Part model, mm, in its own coordinate system. A direction names the side the tool comes from. Coordinates: 2 decimals unless noted, no trailing zeros. Write each loop counter-clockwise with the first axis right and the second up, starting at its lowest first coordinate (ties: lowest second). Pieces come first, ordered by that corner, then holes. Notation, with made-up numbers: (-8.75, 44.25) -> (29.25, 44.25) arc R21 cw to (29.25, 53.25) -> close; hole circle Ø7 at (-37.5, 55.25). An arc over 180 degrees is marked (long way). One line per question, with ' | ' between items. Start each with the question number.
Item 1: Pin check, flat tips, straight feed: pin 1 (2 mm diameter, centred on y = 3.5, z = -2.5, fed in from +X); pin 2 (5 mm diameter, centred on x = 1.5, y = 4.5, fed in from +Z); pin 3 (1.5 mm diameter, centred on y = 2, z = -3.5, fed in from -X); pin 4 (1 mm diameter, centred on y = 4, z = 2.5, fed in from -X). Stop position of each tip, or through.
Item 2: Saw through at B-B (y = 6.75). List the corners of the cut face in (x, z) (1 decimal).
Item 3: Saw through at D-D (x = -3). List the corners of the cut face in (y, z).
Item 4: Two-plate mould, pull along Y, no slides. Class faces 3 (the cylindrical face through (-1.514, 6.887, -0.477)), 4 (the conical face through (-2.09, 3.75, -0.17)), 5 (the flat face through (-1.3, 13.97, -1.3)): pulls with the +Y half, pulls with the -Y half, needs draft (parallel to the pull), parting line crosses it, or undercut.
Item 5: Probe probe 1 along Z at (x, y) = (0, 11); probe 2 along Z at (x, y) = (0.75, 11.25). List the from-to ranges inside material, lowest first. Write a range as [from, to].
Item 6: 3-axis set-ups, long thin cutter, end or side, ignore diameter. For faces 1 (the cylindrical face through (2.807, 4.783, 0.232)), 2 (the cylindrical face through (-4.23, 6.89, 3.25)): which of +Z, -Z, +X, -X, +Y, -Y reach the whole face in a straight line?
Item 7: Saw through at C-C (x = 2). Count the separate pieces of the cut face and the enclosed holes in it, and give its area (3 significant figures).
Item 8: Saw through at A-A (x = 0). List the corners of the cut face in (y, z).
from build123d import *

# Parameters (mm, degrees)
SKETCH1_R           = 5.334
BOSS_EXTRUDE1_DEPTH = 13.97
SKETCH2_R           = 1.5875
CUT_EXTRUDE1_DEPTH  = 14.97


with BuildPart() as part:
    # Sketch1 → Boss-Extrude1 (new body)
    with BuildSketch(Plane(origin=(0, 0, 0), x_dir=(1, 0, 0), z_dir=(0, 1, 0))):
        Circle(SKETCH1_R)
    extrude(amount=BOSS_EXTRUDE1_DEPTH)

    # Sketch2 → Cut-Extrude1 (cut, through all)
    with BuildSketch(Plane(origin=(0, 0, 0), x_dir=(-1, 0, 0), z_dir=(0, -1, 0))):
        Circle(SKETCH2_R)
    extrude(amount=-CUT_EXTRUDE1_DEPTH, mode=Mode.SUBTRACT)

    # Sketch6 → CSK for #2 Flat Head Machine Screw (100)2 (revolve, cut)
    with BuildSketch(Plane(origin=(5.33394419, 3.679102393, -0.024400355), x_dir=(-0.004574495, 0, -0.999989537), z_dir=(0, 1, 0))):
        Polygon((0, 0), (0, 7.537152758), (1.1303, 6.858), (1.1303, 0.884494921), (2.1844, 0), align=None)
    csk_for_2_flat_head_machine_screw_100 = revolve(axis=Axis((11.68387775, 3.679102393, -0.053448397), (-0.999989537, 0, 0.004574495)), mode=Mode.SUBTRACT)

    # Mirror3: CSK for #2 Flat Head Machine Screw (100)2 across plane
    add(csk_for_2_flat_head_machine_screw_100.mirror(Plane(origin=(0, 6.985, 0), x_dir=(0, 0, 1), z_dir=(0, -1, 0))), mode=Mode.SUBTRACT)


solid = part.part
From the geometry:
1) pin 1: x = 5.05 | pin 2: z = 5.33 | pin 3: x = -4.57 | pin 4: x = -4.94
2) outline: circle Ø10.7 at (0, 0); hole circle Ø3.2 at (0, 0)
3) outline: (0, -4.41) -> (13.97, -4.41) -> (13.97, 4.41) -> (0, 4.41) -> close
4) face 3: needs draft | face 4: undercut | face 5: pulls with the +Y half
5) probe 1: [-5.33, -1.59], [1.59, 5.33] | probe 2: [-5.28, -1.4], [1.4, 5.28]
6) face 1: none | face 2: +Y, -Y
7) separate pieces: 1 | enclosed holes: 2 | area: 130 mm2
8) outline: (0, -5.33) -> (13.97, -5.33) -> (13.97, -1.59) -> (0, -1.59) -> close; (0, 1.59) -> (13.97, 1.59) -> (13.97, 5.33) -> (0, 5.33) -> close
